Input: dimensioned drawing with shaded views. Units: mm. Origin: part minimum x, y, z. Round coordinates to 2 decimals unless told otherwise and drop trailing zeros. Write each loop counter-clockwise with the first axis right and the second up, starting at its lowest first coordinate (ties: lowest second). Pieces come first, ordered by that corner, then holes. Notation, with made-up numbers: (27.25, 38) -> (63.25, 38) arc R29 ccw to (63.25, 74) -> close; hole circle Ø1 at (17.25, -36.75). An arc over 180 degrees is marked (long way). Return JSON: item names as keys, results as strings. Group by question number.
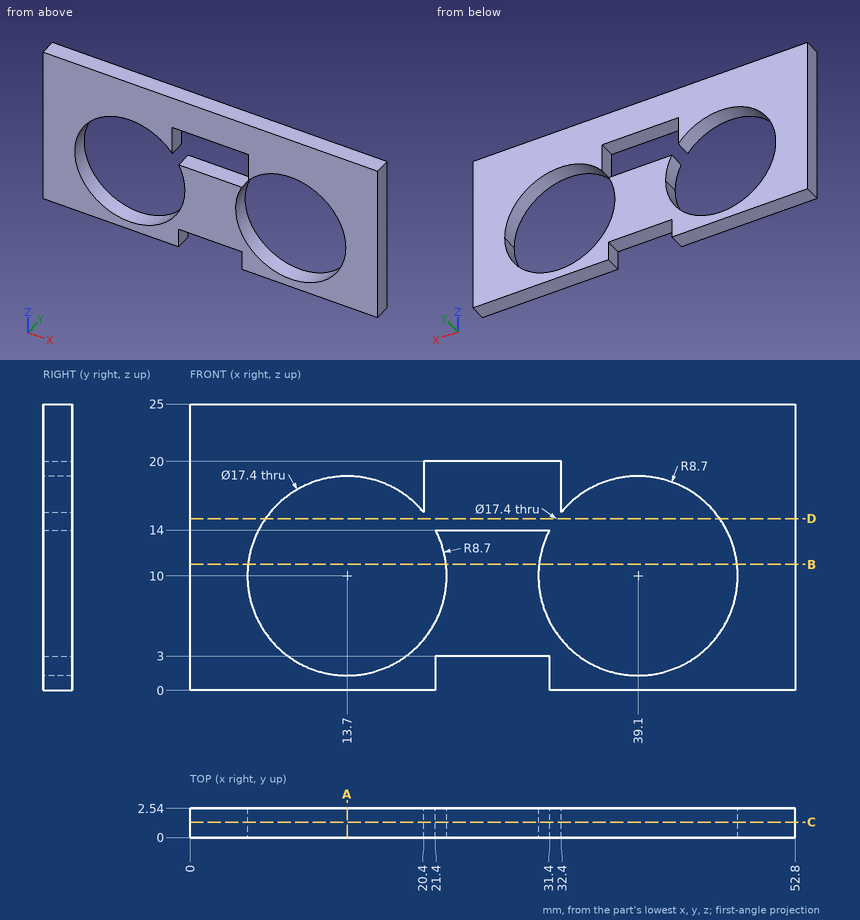
Item 1: Cut plane A-A on x = 13.7. Output: boundary loops of the cut face in (y, z), and give its area (3 significant figures).
Item 2: Cut plane C-C on y = 1.35. Output: boundary loops of the cut face in (x, z), and give its area (3 significant figures).
Item 3: Cut plane B-B on z = 11. Output: boundary loops of the cut face in (x, y), and give its area (3 significant figures).
Item 4: Cut plane D-D on z = 15. Output: boundary loops of the cut face in (x, y), and give its area (3 significant figures).
Item 5: Material intervals for probe 1 along X at (y, z) = (1.95, 10); probe 2 along Z at (x, y) = (13.7, 1.6); probe 3 along Z at (x, y) = (25.5, 1.2), sorted ascending.
Item 6: First-contact query: pin 1 Ø4 at (x, z) = (7, 11) entering from +Y; pin 2 Ø1.3 at (x, y) = (29, 1.5) entering from -Z; pin 3 Ø3 at (x, z) = (33, 8) entering from -Y. Flat tips, straight axial feed; report the tip coordinate or a pass-through.
Here are the results:
{
 "1": {"outline": "(0, 0) -> (2.54, 0) -> (2.54, 1.3) -> (0, 1.3) -> close; (0, 18.7) -> (2.54, 18.7) -> (2.54, 25) -> (0, 25) -> close", "area": "19.3 mm^2"},
 "2": {"outline": "(0, 0) -> (21.4, 0) -> (21.4, 3) -> (31.4, 3) -> (31.4, 0) -> (52.8, 0) -> (52.8, 25) -> (0, 25) -> close; hole (20.4, 15.55) arc R8.7 ccw (long way) to (21.43, 14) -> (31.37, 14) arc R8.7 ccw (long way) to (32.4, 15.55) -> (32.4, 20) -> (20.4, 20) -> close", "area": "744 mm^2"},
 "3": {"outline": "(0, 0) -> (5.06, 0) -> (5.06, 2.54) -> (0, 2.54) -> close; (22.34, 0) -> (30.46, 0) -> (30.46, 2.54) -> (22.34, 2.54) -> close; (47.74, 0) -> (52.8, 0) -> (52.8, 2.54) -> (47.74, 2.54) -> close", "area": "46.3 mm^2"},
 "4": {"outline": "(0, 0) -> (6.58, 0) -> (6.58, 2.54) -> (0, 2.54) -> close; (46.22, 0) -> (52.8, 0) -> (52.8, 2.54) -> (46.22, 2.54) -> close", "area": "33.4 mm^2"},
 "5": {"probe 1": "x = 0 to 5, 22.4 to 30.4, 47.8 to 52.8", "probe 2": "z = 0 to 1.3, 18.7 to 25", "probe 3": "z = 3 to 14, 20 to 25"},
 "6": {"pin 1": "stops at y = 2.54", "pin 2": "stops at z = 3", "pin 3": "passes through"}
}
